from build123d import *

# Parameters (mm, degrees)
F0_R     = 11
F1_DEPTH = 5
F2_SIZE2 = 0.5
F2_SIZE  = 0.5
F3_SIZE2 = 0.5
F3_SIZE  = 0.5


with BuildPart() as f1:
    # F0 (on Top) → F1 (new body, symmetric)
    with BuildSketch(Plane.XY):
        with BuildLine():
            Line((-16.026402, 13.960794), (-7.816408, 13.960794))
            ThreePointArc((-7.816408, 13.960794), (-15.997645, 0.274512), (-8.290786, -13.684402))
            Line((-8.290786, -13.684402), (-16.026402, -13.684402))
            Line((-16.026402, -13.684402), (-16.026402, -20.231948))
            Line((-16.026402, -20.231948), (15.973598, -20.231948))
            Line((15.973598, -20.231948), (15.973598, -13.684402))
            Line((15.973598, -13.684402), (8.290786, -13.684402))
            ThreePointArc((8.290786, -13.684402), (15.997645, 0.274512), (7.816408, 13.960794))
            Line((7.816408, 13.960794), (15.973598, 13.960794))
            Line((15.973598, 13.960794), (15.973598, 20.50834))
            Line((15.973598, 20.50834), (-16.026402, 20.50834))
            Line((-16.026402, 20.50834), (-16.026402, 13.960794))
        make_face()
        Circle(F0_R, mode=Mode.SUBTRACT)
    extrude(amount=F1_DEPTH, both=True)

    # F2
    f2_edges = [f1.edges().sort_by_distance(p)[0] for p in [
        (15.973598, 17.234567, 5),
        (-0.026402, 20.50834, 5),
        (-16.026402, 17.234567, 5),
        (-11.921405, 13.960794, 5),
        (-15.997645, 0.274512, 5),
        (-12.158594, -13.684402, 5),
        (-16.026402, -16.958175, 5),
        (-0.026402, -20.231948, 5),
        (15.973598, -16.958175, 5),
        (12.132192, -13.684402, 5),
        (15.997645, 0.274512, 5),
        (11.895003, 13.960794, 5),
        (-11, 0, 5),
    ]]
    chamfer(f2_edges, length=F2_SIZE, length2=F2_SIZE2)

    # F3
    f3_edges = [f1.edges().sort_by_distance(p)[0] for p in [
        (15.973598, 17.234567, -5),
        (-0.026402, 20.50834, -5),
        (-16.026402, 17.234567, -5),
        (-11.921405, 13.960794, -5),
        (-15.997645, 0.274512, -5),
        (-12.158594, -13.684402, -5),
        (-16.026402, -16.958175, -5),
        (-0.026402, -20.231948, -5),
        (15.973598, -16.958175, -5),
        (12.132192, -13.684402, -5),
        (15.997645, 0.274512, -5),
        (11.895003, 13.960794, -5),
        (-11, 0, -5),
    ]]
    chamfer(f3_edges, length=F3_SIZE, length2=F3_SIZE2)


solid = f1.part
Source: CAD feature listing. Evaluate the final solid. Frame: model axes, mm. A direction names the side the tool comes from. Coordinates: 2 decimals unless noted, no trailing zeros. Loops run counter-clockwise (first coordinate to the right, second up) from the corner with the lowest first, then second, coordinate; pieces in that order, holes last. Notation, with made-up numbers: (45, 30) -> (70, 30) arc R8 ccw to (70, 38) -> close; hole circle Ø8 at (25, 68.5). An arc over 180 degrees is marked (long way). Answer in a Markdown table with one row per item. Add a question column.
Q1. Section B-B on x = 0. Return the cut outline in (y, z).
Q2. Ray query, line 1 along Y through (x, z) = (-11.5, 4); line 2 along Y through (x, z) = (0, 0); line 3 along Y through (x, z) = (9.5, 2.5). Return the intervals inside material, ascending.
Q3. Reachability of faces 5 (the face through (-12, 13.961, 0)), 6 (the face through (12, -13.684, 0)), 7 (the face through (-7.13, 9.25, 5)) from +Z, -Z, +X, -X, +Y, -Y: full face, straight path, thin tool, end or side. Return the list, or none.
Q4. Pull-direction query (Y, two-part tool) for faces 1 (the face through (0, 20.508, 0)), 2 (the face through (-16.026, 17, 0)), 3 (the face through (0, -20.232, 0)), 4 (the face through (-15.63, 0.62, 4.86)); classes: pulls with the +Y half, pulls with the -Y half, needs draft (parallel to the pull), parting line crosses it, or undercut.
Q5. Section A-A on y = 0. Return the cut outline in (x, z), and give its area (3 significant figures).
Q6. Section D-D on x = 14.5. Give the number of separate pieces and of enclosed holes in the cut face, and give its area (3 significant figures).
Q7. Section C-C on z = 0.75. Return the cut outline in (x, y), and give its area (3 significant figures).
Q8. Contact query for flat-ended pins moving along their axis: pin 1 Ø5 at (y, z) = (17, 1.5) entering from +X; pin 2 Ø13 at (x, y) = (0, 0) entering from -Z; pin 3 Ø3 at (y, z) = (-11, 2.5) entering from -X. Output: stop coordinate, or through.
Computed values:
| question | item | result |
|---|---|---|
| 1 | outline | (-20.23, -4.5) -> (-19.73, -5) -> (-11.5, -5) -> (-11, -4.5) -> (-11, 4.5) -> (-11.5, 5) -> (-19.73, 5) -> (-20.23, 4.5) -> close; (11, -4.5) -> (11.5, -5) -> (20.01, -5) -> (20.51, -4.5) -> (20.51, 4.5) -> (20.01, 5) -> (11.5, 5) -> (11, 4.5) -> close |
| 2 | line 1 | y = -20.23 to -13.68, -11.12 to 11.12, 13.96 to 20.51 |
| 2 | line 2 | y = -20.23 to -11, 11 to 20.51 |
| 2 | line 3 | y = -20.23 to -13.68, -12.87 to -5.55, 5.55 to 12.87, 13.96 to 20.51 |
| 3 | face 5 | +Z, -Z, -X |
| 3 | face 6 | +Z, -Z, +X |
| 3 | face 7 | +Z, +X, -X, +Y, -Y |
| 4 | face 1 | pulls with the +Y half |
| 4 | face 2 | needs draft |
| 4 | face 3 | pulls with the -Y half |
| 4 | face 4 | undercut |
| 5 | outline | (-16, -4.5) -> (-15.5, -5) -> (-11.5, -5) -> (-11, -4.5) -> (-11, 4.5) -> (-11.5, 5) -> (-15.5, 5) -> (-16, 4.5) -> close; (11, -4.5) -> (11.5, -5) -> (15.5, -5) -> (16, -4.5) -> (16, 4.5) -> (15.5, 5) -> (11.5, 5) -> (11, 4.5) -> close |
| 5 | area | 99.0 mm^2 |
| 6 | separate pieces | 3 |
| 6 | enclosed holes | 0 |
| 6 | area | 264 mm^2 |
| 7 | outline | (-16.03, -20.23) -> (15.97, -20.23) -> (15.97, -13.68) -> (8.29, -13.68) arc R16 ccw to (7.82, 13.96) -> (15.97, 13.96) -> (15.97, 20.51) -> (-16.03, 20.51) -> (-16.03, 13.96) -> (-7.82, 13.96) arc R16 ccw to (-8.29, -13.68) -> (-16.03, -13.68) -> close; hole circle Ø22 at (0, 0) |
| 7 | area | 796 mm^2 |
| 8 | pin 1 | stops at x = 15.97 |
| 8 | pin 2 | passes through |
| 8 | pin 3 | stops at x = -12.87 |
